from build123d import *


with BuildPart() as part:
    # Sketch1 → Revolve1 (revolve)
    with BuildSketch(Plane.XY):
        with BuildLine():
            Line((0, 0), (-80.5, 0))
            add(Edge.make_bspline(
                [(-74, 2), (-80.5, 2), (-80.5, 0)],
                knots=[4.71238898, 4.71238898, 4.71238898, 6.283185307, 6.283185307, 6.283185307], degree=2, weights=[1, 0.707106781, 1]))
            Line((-74, 2), (-74, 3.05))
            Line((-74, 3.05), (-69, 3.05))
            ThreePointArc((-69, 3.05), (-66.68703246, 4.51758115), (-64, 5.05))
            Line((-64, 5.05), (-50, 5.2))
            Line((-50, 5.2), (-50, 6.325))
            add(Edge.make_bspline(
                [(-50, 6.325), (-26.936405274, 6.325), (-9.347344877, 6.218788302), (-5.5, 5.1)],
                knots=[0, 0, 0, 0, 0.970469824, 0.970469824, 0.970469824, 0.970469824], degree=3))
            Line((-5.5, 5.1), (-0.720771547, 3.710224698))
            ThreePointArc((-0.720771547, 3.710224698), (-0.200241145, 3.350321392), (0, 2.75))
            Line((0, 2.75), (0, 0))
        make_face()
    revolve(axis=Axis((0, 0, 0), (-1, 0, 0)))


solid = part.part
Source: CAD feature listing. Evaluate the final solid. Frame: model axes, mm. A direction names the side the tool comes from. Round coordinates to 2 decimals unless told otherwise and drop trailing zeros. Loops run counter-clockwise (first coordinate to the right, second up) from the corner with the lowest first, then second, coordinate; pieces in that order, holes last. Notation, with made-up numbers: M -26,10.25 L 2,10.25 A25 cw 2,28.25 Z; hole C -27,72.5 d3. An arc over 180 degrees is marked long. Return JSON: item names as keys, results as strings. Group by question number.
1. Section query A-A on x = -71.5. Output: boundary loops of the cut face in (y, z), and give its area (3 significant figures).
2. Material intervals for line 1 along Z through (x, y) = (-54.5, -4.75); line 2 along Y through (x, z) = (-27, -5); line 3 along Y through (x, z) = (-66.5, 0.75), sorted ascending. Write a range as from..to.
3. Section query B-B on x = -51.5. Output: boundary loops of the cut face in (y, z).
4. Reachability of faces 1 (the face through (0, 0, 0)), 2 (the face through (-71.465, -3.047, -0.134)) from +Z, -Z, +X, -X, +Y, -Y: full face, straight path, thin tool, end or side. Return the list, or none.
5. Pin query (flat end, axial travel): pin 1 (4 mm diameter, centred on x = -8, y = -2.5, fed in from -Z); pin 2 (6 mm diameter, centred on x = -23.5, y = -2.5, fed in from -Z); pin 3 (4 mm diameter, centred on y = -1, z = -4, fed in from -X). Return the tip coordinate at first contact, or that it passes through.
Checks:
{
 "1": {"outline": "C 0,0 d6.1", "area": "29.2 mm²"},
 "2": {"line 1": "z = -1.99..1.99", "line 2": "y = -3.72..3.72", "line 3": "y = -4.53..4.53"},
 "3": {"outline": "C 0,0 d10.37"},
 "4": {"face 1": "+Z, -Z, +X, +Y, -Y", "face 2": "-X"},
 "5": {"pin 1": "stops at z = -5.57", "pin 2": "stops at z = -6.21", "pin 3": "stops at x = -74"}
}
